from build123d import *

# Parameters (mm, degrees)
PAD015_DEPTH    = 12
SKETCH032_R     = 1.5
POCKET013_DEPTH = 25.001
SKETCH034_R     = 2.55
POCKET014_DEPTH = 25.001
POCKET015_DEPTH = 15
POCKET016_DEPTH = 4
FILLET_R        = 5


with BuildPart() as part:
    # Sketch029 → Pad015 (new body)
    with BuildSketch(Plane.XZ):
        Polygon((77.4690929999, 0), (77.4690929999, -25), (-24.29069, -25), (-24.29069, -15), (38.3828349999, -15), (38.3828349999, 0), (49.7345464999, 0), (49.7345464999, -7.5), (61.7345464999, -7.5), (61.7345464999, 0), align=None)
    extrude(amount=PAD015_DEPTH)

    # Sketch032 → Pocket013 (cut, through all)
    with BuildSketch(Plane.XY):
        with Locations((44.8828349999, -6)):
            Circle(SKETCH032_R)
        with Locations((66.586258, -6)):
            Circle(SKETCH032_R)
    extrude(amount=-POCKET013_DEPTH, mode=Mode.SUBTRACT)

    # Sketch034 → Pocket014 (cut, through all)
    with BuildSketch(Plane.XY):
        with Locations((-5.7879446208, -6)):
            Circle(SKETCH034_R)
        with Locations((20.4831280675, -6)):
            Circle(SKETCH034_R)
    extrude(amount=-POCKET014_DEPTH, mode=Mode.SUBTRACT)

    # Sketch035 (on Face3 of Pocket014) → Pocket015 (cut)
    with BuildSketch(Plane(origin=(0, 0, -25), x_dir=(1, 0, 0), z_dir=(0, 0, -1))):
        Polygon((46.586018294, 8.95), (43.1796517057, 8.95), (41.4764684116, 6), (43.1796517057, 3.05), (46.586018294, 3.05), (48.2892015881, 6), align=None)
        Polygon((68.2894412941, 8.95), (64.8830747059, 8.95), (63.1798914118, 6), (64.8830747059, 3.05), (68.2894412941, 3.05), (69.9926245882, 6), align=None)
    extrude(amount=-POCKET015_DEPTH, mode=Mode.SUBTRACT)

    # Sketch036 (on Face23 of Pocket015) → Pocket016 (cut)
    with BuildSketch(Plane(origin=(0, 0, -15), x_dir=(-1, 0, 0), z_dir=(0, 0, 1))):
        Polygon((-22.9368667116, 10.25), (-25.3906053556, 6), (-22.9368667116, 1.75), (-18.0293894234, 1.75), (-15.5756507794, 6), (-18.0293894234, 10.25), align=None)
        Polygon((3.3342059768, 10.25), (0.8804673327, 6), (3.3342059768, 1.75), (8.2416832649, 1.75), (10.6954219089, 6), (8.2416832649, 10.25), align=None)
    extrude(amount=-POCKET016_DEPTH, mode=Mode.SUBTRACT)

    # Fillet
    fillet_edges = [part.edges().sort_by_distance(p)[0] for p in [
        (77.469093, -6, -25),
    ]]
    fillet(fillet_edges, radius=FILLET_R)


with BuildPart() as part_1:
    # Body005 placement: moved
    add(part.part.moved(Location((0, 29, -22))))


solid = part_1.part
The listing builds one solid part. Answer for the finished solid, in the listing's coordinates (mm). A direction names the side the tool comes from. Give positions to 0.01 mm unless a question says otherwise; leave off trailing zeros. Loops run counter-clockwise (first coordinate to the right, second up) from the corner with the lowest first, then second, coordinate; pieces in that order, holes last. Notation, with made-up numbers: (50.25, 84.25) - (106.25, 84.25) arc R24 ccw to (106.25, 94.25) - close; hole circle Ø1 at (14.25, 19.25). An arc over 180 degrees is marked (long way). Write each question's results on one line, items separated by ' | '.
1. Which of the six approach directions +Z, -Z, +X, -X, +Y, -Y give full straight-line access (tool end or side, diameter ignored) to faces 1 (the face through (64.043, 21.504, -39.605)), 2 (the face through (49.735, 23, -26)), 3 (the face through (-9.451, 25.155, -38.972)), 4 (the face through (7, 23, -37))?
Resolved:
face 1: -Z | face 2: +Z, +Y, -Y | face 3: +Z | face 4: +Z, -X, +Y, -Y
2. Flat-ended cylindrical pins translate along their axes: P1, Ø4, axis at x = 66.59, y = 23, coming from the -Z side; P2, Ø6, axis at y = 23.5, z = -27, coming from the -X side; P3, Ø3.5, axis at x = 8.5, y = 22.5, coming from the +Z side; P4, Ø4.5, axis at x = 20.48, y = 23, coming from the -Z side. Find the tip coordinate at first contact, or state that the pin passes through.
Resolved:
P1: stops at z = -32 | P2: stops at x = 38.38 | P3: stops at z = -37 | P4: passes through
3. Find section B-B, the plane z = -33.5. Write down the section's boundary in (x, y).
Resolved:
outline: (38.38, 17) - (77.47, 17) - (77.47, 29) - (38.38, 29) - close; hole (41.48, 23) - (43.18, 20.05) - (46.59, 20.05) - (48.29, 23) - (46.59, 25.95) - (43.18, 25.95) - close; hole (63.18, 23) - (64.88, 20.05) - (68.29, 20.05) - (69.99, 23) - (68.29, 25.95) - (64.88, 25.95) - close
4. Find section A-A, the plane z = -26.5. Write down the section's boundary in (x, y), then the cut area to 3 significant figures.
Resolved:
outline: (38.38, 17) - (49.73, 17) - (49.73, 29) - (38.38, 29) - close; (61.73, 17) - (77.47, 17) - (77.47, 29) - (61.73, 29) - close; hole circle Ø3 at (44.88, 23); hole circle Ø3 at (66.59, 23) | area: 311 mm^2
5. For a pull along X with two mould halves and no side action, classify faces 5 (the face through (77.469, 23, -32)), 6 (the face through (25, 23, -47)), 7 (the face through (42.34, 21.504, -39.605)) as +X half, -X half, draft (parallel to the pull), parting line (faces both ways), or undercut.
Resolved:
face 5: +X half | face 6: draft | face 7: undercut
6. Find section C-C, the plane x = 19.5. Write down the section's boundary in (y, z), then the cut area to 3 significant figures.
Resolved:
outline: (17, -47) - (20.65, -47) - (20.65, -41) - (18.75, -41) - (18.75, -37) - (17, -37) - close; (25.35, -47) - (29, -47) - (29, -37) - (27.25, -37) - (27.25, -41) - (25.35, -41) - close | area: 57.8 mm^2
7. Consider probe 1 along X at (y, z) = (23, -38.5); probe 2 along Y at (x, z) = (-5, -38); probe 3 along X at (y, z) = (19.25, -25). Determine where each line is inside the solid, lowest interval first. Write a range as from..to.
Resolved:
probe 1: x = -24.29..-10.7, -0.88..15.58, 25.39..41.48, 48.29..63.18, 69.99..77.47 | probe 2: y = 17..18.75, 27.25..29 | probe 3: x = 38.38..49.73, 61.73..77.47
